Source: CAD feature listing. Evaluate the final solid. Frame: model axes, mm. A direction names the side the tool comes from. Round coordinates to 2 decimals unless told otherwise and drop trailing zeros. Loops run counter-clockwise (first coordinate to the right, second up) from the corner with the lowest first, then second, coordinate; pieces in that order, holes last. Notation, with made-up numbers: (44.25, -27.5) - (57.25, -27.5) arc R17 cw to (57.25, -18.5) - close; hole circle Ø7 at (71, -9.5). An arc over 180 degrees is marked (long way). Use CSV: the item, a comma, the result in double quotes. Start each with the question number.
from build123d import *

# Parameters (mm, degrees)
BOSS_EXTRU_1_DEPTH = 15


with BuildPart() as part:
    # Esquisse1 → Boss.-Extru.1 (new body)
    with BuildSketch(Plane.XY):
        with BuildLine():
            Line((65, 37.5), (-65, 37.5))
            ThreePointArc((-65, 37.5), (-72.071067812, 34.571067812), (-75, 27.5))
            Line((-75, 27.5), (-75, -27.5))
            ThreePointArc((-75, -27.5), (-72.071067812, -34.571067812), (-65, -37.5))
            Line((-65, -37.5), (-60, -37.5))
            Line((-60, -37.5), (-60, -22.5))
            Line((-60, -22.5), (-55, -22.5))
            Line((-55, -22.5), (-55, -13.973661668))
            Line((-55, -13.973661668), (-62.5, -13.973661668))
            Line((-62.5, -13.973661668), (-62.5, -5.973661668))
            Line((-62.5, -5.973661668), (-55, -5.973661668))
            Line((-55, -5.973661668), (-55, 2.552676663))
            Line((-55, 2.552676663), (-45, 2.552676663))
            Line((-45, 2.552676663), (-45, -5.973661668))
            Line((-45, -5.973661668), (-37.5, -5.973661668))
            Line((-37.5, -5.973661668), (-37.5, -13.973661668))
            Line((-37.5, -13.973661668), (-45, -13.973661668))
            Line((-45, -13.973661668), (-45, -22.5))
            Line((-45, -22.5), (-27.5, -22.5))
            Line((-27.5, -22.5), (-27.5, -7.5))
            Line((-27.5, -7.5), (-7.5, -7.5))
            Line((-7.5, -7.5), (-7.5, 15))
            Line((-7.5, 15), (7.5, 15))
            Line((7.5, 15), (7.5, -7.5))
            Line((7.5, -7.5), (27.5, -7.5))
            Line((27.5, -7.5), (27.5, -22.5))
            Line((27.5, -22.5), (45, -22.5))
            Line((45, -22.5), (45, -13.973661668))
            Line((45, -13.973661668), (37.5, -13.973661668))
            Line((37.5, -13.973661668), (37.5, -5.973661668))
            Line((37.5, -5.973661668), (45, -5.973661668))
            Line((45, -5.973661668), (45, 2.552676663))
            Line((45, 2.552676663), (55, 2.552676663))
            Line((55, 2.552676663), (55, -5.973661668))
            Line((55, -5.973661668), (62.5, -5.973661668))
            Line((62.5, -5.973661668), (62.5, -13.973661668))
            Line((62.5, -13.973661668), (55, -13.973661668))
            Line((55, -13.973661668), (55, -22.5))
            Line((55, -22.5), (60, -22.5))
            Line((60, -22.5), (60, -37.5))
            Line((60, -37.5), (65, -37.5))
            ThreePointArc((65, -37.5), (72.071067812, -34.571067812), (75, -27.5))
            Line((75, -27.5), (75, 27.5))
            ThreePointArc((75, 27.5), (72.071067812, 34.571067812), (65, 37.5))
        make_face()
    extrude(amount=BOSS_EXTRU_1_DEPTH)


solid = part.part
1. Section query B-B on y = 1. Return the cut outline in (x, z).
2. Section query D-D on y = -25. Return the cut outline in (x, z), and give its area (3 significant figures).
3. Contact query for flat-ended pins moving along their axis: P1, Ø6, axis at x = 45.5, y = 29, coming from the -Z side; P2, Ø7.5, axis at x = -2, z = 6, coming from the -Y side; P3, Ø2, axis at x = 42.5, z = 4.5, coming from the -Y side; P4, Ø4.5, axis at x = -20.5, z = 4.5, coming from the -Y side. Output: stop coordinate, or through.
4. Reachability of faces 1 (the flat face through (-41, -13.974, 7)), 2 (the flat face through (62, -37.5, 7)), 3 (the flat face through (45, -2, 7)) from +Z, -Z, +X, -X, +Y, -Y: full face, straight path, thin tool, end or side. Return the list, or none.
5. Section query A-A on y = 9.5. Return the cut outline in (x, z), and give its area (4 significant figures).
6. Mould query, pull axis X, two halves, no side actions, for faces 4 (the flat face through (1, 37.5, 7)), 5 (the cylindrical face through (72.15, 34.49, 7.4)), 6 (the flat face through (60, -30, 7)). Classes: +X half, -X half, draft (parallel to the pull), parting line (faces both ways), or undercut.
7. Line query: line 1 along X through (y, z) = (-26, 14.75); line 2 along X through (y, z) = (7.5, 12); line 3 along Y through (x, z) = (42.5, 1.5). Output: solid intervals per line, ascending.
8. Section query C-C on x = -15. Return the cut outline in (y, z).
Values:
1,outline,"(-75, 0) - (-55, 0) - (-55, 15) - (-75, 15) - close; (-45, 0) - (-7.5, 0) - (-7.5, 15) - (-45, 15) - close; (7.5, 0) - (45, 0) - (45, 15) - (7.5, 15) - close; (55, 0) - (75, 0) - (75, 15) - (55, 15) - close"
2,outline,"(-75, 0) - (-60, 0) - (-60, 15) - (-75, 15) - close; (60, 0) - (75, 0) - (75, 15) - (60, 15) - close"
2,area,"450 mm^2"
3,P1,"stops at z = 0"
3,P2,"stops at y = 15"
3,P3,"stops at y = -22.5"
3,P4,"stops at y = -7.5"
4,face 1,"+Z, -Z"
4,face 2,"+Z, -Z, +X, -X, -Y"
4,face 3,"+Z, -Z, -Y"
5,outline,"(-75, 0) - (-7.5, 0) - (-7.5, 15) - (-75, 15) - close; (7.5, 0) - (75, 0) - (75, 15) - (7.5, 15) - close"
5,area,"2,025 mm^2"
6,face 4,"draft"
6,face 5,"+X half"
6,face 6,"undercut"
7,line 1,"x = -75 to -60, 60 to 75"
7,line 2,"x = -75 to -7.5, 7.5 to 75"
7,line 3,"y = -22.5 to -13.97, -5.97 to 37.5"
8,outline,"(-7.5, 0) - (37.5, 0) - (37.5, 15) - (-7.5, 15) - close"
